Here's how the part is built. I have some questions about the finished solid (model axes, mm). A direction names the side the tool comes from. Give positions to 0.01 mm unless a question says otherwise; leave off trailing zeros. Write each loop counter-clockwise with the first axis right and the second up, starting at its lowest first coordinate (ties: lowest second). Pieces come first, ordered by that corner, then holes. Notation, with made-up numbers: (39, 28.5) -> (59, 28.5) arc R25 ccw to (59, 55.5) -> close; hole circle Ø1 at (41, 2.5). An arc over 180 degrees is marked (long way). Use one line per item in the form item = value.
```python
from build123d import *

# Parameters (mm, degrees)
SKETCH_1_R             = 12.5
EXTRUDE_1_DEPTH        = 60
HOLE_WIZARD_M6_1_D     = 5
HOLE_WIZARD_M6_1_DEPTH = 15
HOLE_WIZARD_M6_1_TIP   = 1.502151548
CHAMFER_1_SIZE         = 0.2


with BuildPart() as part:
    # 草图1 → 凸台-拉伸1 (new body)
    with BuildSketch(Plane(origin=(0, 0, 0), x_dir=(1, 0, 0), z_dir=(0, 1, 0))):
        with Locations(Location((0, 0, 0), (0, 0, 270))):
            Circle(SKETCH_1_R)
    extrude(amount=EXTRUDE_1_DEPTH)

    # M6 螺纹孔1
    with Locations(Plane(origin=(0, 60, 0), x_dir=(1, 0, 0), z_dir=(0, 1, 0))):
        with Locations((0, 0)):
            Hole(HOLE_WIZARD_M6_1_D / 2, depth=HOLE_WIZARD_M6_1_DEPTH)
            with Locations((0, 0, -(HOLE_WIZARD_M6_1_DEPTH + HOLE_WIZARD_M6_1_TIP / 2))):  # 118° drill point
                Cone(0, HOLE_WIZARD_M6_1_D / 2, HOLE_WIZARD_M6_1_TIP, mode=Mode.SUBTRACT)

    # 倒角1
    chamfer_1_edges = [part.edges().sort_by_distance(p)[0] for p in [
        (0, 0, -12.5),
        (0, 60, -12.5),
    ]]
    chamfer(chamfer_1_edges, length=CHAMFER_1_SIZE)


solid = part.part
```
Q1. I want a section at A-A, the plane y = 50. Write out the boundary of the cut face in (x, z).
Result set:
outline = circle Ø25 at (0, 0); hole circle Ø5 at (0, 0)
Q2. If I drill on line 1 along Z through (x, y) = (-0.5, 7.5); line 2 along Z through (x, y) = (-0.5, 57); line 3 along Z through (x, y) = (-2.25, 4.5), over which ranges is the centre line in solid material (lowest first)? Write a range as from..to.
Result set:
line_1 = -12.49..12.49
line_2 = -12.49..-2.45, 2.45..12.49
line_3 = -12.3..12.3
Q3. Which directions (+Z, -Z, +X, -X, +Y, -Y) give clear straight access to the entire face, cutting with the end or side of a thin tool? Please do faces 4 (the face through (0.54, 52.4, 2.44)), 5 (the face through (0, 60, 3)).
Result set:
face_4 = +Y
face_5 = +Z, -Z, +X, -X, +Y
Q4. I want a section at B-B, the plane y = 16. Write out the boundary of the cut face in (x, z).
Result set:
outline = circle Ø25 at (0, 0)
Q5. If we mould it in two halves opening along X, with no side actions, what happens to faces 1 (the face through (0, 0, 0)), 2 (the face through (-0.094, 43.759, 0.424)), 3 (the face through (3.755, 29.583, 11.923))? For each: +X half, -X half, draft (parallel to the pull), parting line (faces both ways), or undercut.
Result set:
face_1 = draft
face_2 = undercut
face_3 = parting line
Q6. Will these pins go through, and if not, where does the flat tip stop? pin 1 Ø5 at (x, y) = (5.5, 13) entering from -Z; pin 2 Ø3 at (x, z) = (0, 0) entering from +Y; pin 3 Ø2 at (y, z) = (43, 3.5) entering from -X.
Result set:
pin_1 = -12.13
pin_2 = 44.4
pin_3 = -12.25
